Part model, mm, in its own coordinate system. A direction names the side the tool comes from. Round coordinates to 2 decimals unless told otherwise and drop trailing zeros. Loops run counter-clockwise (first coordinate to the right, second up) from the corner with the lowest first, then second, coordinate; pieces in that order, holes last. Notation, with made-up numbers: (30, 2) -> (55, 2) arc R16 cw to (55, 22) -> close; hole circle Ø3 at (3, 51.5). An arc over 180 degrees is marked (long way). Use a Markdown table: item, result. Add a question column.
Item 1: Two-plate mould, pull along Z, no slides. Class faces 3 (the face through (-16, 0, 16)), 4 (the face through (-8.94, -3.76, 20.16)), 5 (the face through (-9.996, -3.757, 2.274)): pulls with the +Z half, pulls with the -Z half, needs draft (parallel to the pull), parting line crosses it, or undercut.
Item 2: Flat gauge pins, fed straight in: pin 1 (0.6 mm diameter, centred on y = -5, z = 21.5, fed in from -X); pin 2 (2 mm diameter, centred on x = -19, y = -3.5, fed in from -Z); pin 3 (4 mm diameter, centred on x = -13.5, y = -5.5, fed in from +Z). Where does each tip first touch, or does it go through?
Item 3: Probe line 1 (X direction, y = -6, z = 18); line 2 (Z direction, x = -17.75, y = -2); line 3 (X direction, y = -5.75, z = 8.5). List the from-to ranges inside material, lowest first. Write a range as [from, to].
Item 4: Cut at C-C, the plane z = 10. List the corners of the cut face in (x, y).
Item 5: Which spindle directions (+Z, -Z, +X, -X, +Y, -Y) get a long thin tool onto all of the face, cutting with end or side? Do faces 1 (the face through (-2.32, -3.76, 9.83)), 2 (the face through (-12.346, -4, 21)). Say none if no direction does.
Item 6: Cut at D-D, the plane z = 18.25. List the corners of the cut face in (x, y), plus the area to 3 significant figures.
Item 7: Cut at B-B, the plane x = -7. List the corners of the cut face in (y, z), plus the area to 3 significant figures.
Item 8: Cut at A-A, the plane y = -2. List the corners of the cut face in (x, z).
```python
from build123d import *

# Parameters (mm, degrees)
F1_DEPTH = 7.62
F3_DEPTH = 7.62
F5_DEPTH = 7.62


with BuildPart() as f1:
    # F0 (on Front) → F1 (new body)
    with BuildSketch(Plane.XZ):
        Polygon((-0.68674681, 15.9189414907), (-9.4810585093, 24.71325319), (-21.4943116993, 21.4943116993), (-24.71325319, 9.4810585093), (-15.9189414907, 0.68674681), (-3.9056883007, 3.9056883007), align=None)
    extrude(amount=F1_DEPTH)

    # F2 (on face) → F3 (cut)
    with BuildSketch(Plane(origin=(0, 0, 0), x_dir=(-1, 0, 0), z_dir=(0, 1, 0))):
        with BuildLine():
            Line((13.7354055899, 8.8358137319), (11.6645944101, 16.5641862681))
            ThreePointArc((11.6645944101, 16.5641862681), (8.8358137319, 11.6645944101), (13.7354055899, 8.8358137319))
        make_face()
        with BuildLine():
            ThreePointArc((16.7005, 12.7), (15.1353500967, 15.8738100378), (11.6645944101, 16.5641862681))
            Line((11.6645944101, 16.5641862681), (13.7354055899, 8.8358137319))
            ThreePointArc((13.7354055899, 8.8358137319), (15.8738100378, 10.2646499033), (16.7005, 12.7))
        make_face()
    extrude(amount=-F3_DEPTH, mode=Mode.SUBTRACT)

    # F4 (on face) → F5 (cut)
    with BuildSketch(Plane(origin=(0, 0, 0), x_dir=(-1, 0, 0), z_dir=(0, 1, 0))):
        with BuildLine():
            Line((9.4810585093, 19.3075097995), (8.38471647, 21.0305488332))
            ThreePointArc((8.38471647, 21.0305488332), (3.6253777463, 10.3186250274), (13.0313017042, 3.323969124))
            Line((13.0313017042, 3.323969124), (13.1753263628, 5.3655037719))
            ThreePointArc((13.1753263628, 5.3655037719), (5.5953016242, 10.8174402904), (9.4810585093, 19.3075097995))
        make_face()
        with BuildLine():
            ThreePointArc((17.3331181487, 4.5419406703), (20.808239175, 7.9802358864), (22.0818823168, 12.7))
            ThreePointArc((22.0818823168, 12.7), (19.2078073532, 19.4578220797), (12.3464885615, 22.0752197558))
            Line((12.3464885615, 22.0752197558), (12.3464885615, 20.0413758747))
            ThreePointArc((12.3464885615, 20.0413758747), (17.7706263223, 18.0206690154), (20.0498823168, 12.7))
            ThreePointArc((20.0498823168, 12.7), (18.9642836617, 8.8555858343), (16.0281797534, 6.1468336203))
            Line((16.0281797534, 6.1468336203), (17.3331181487, 4.5419406703))
        make_face()
    extrude(amount=-F5_DEPTH, mode=Mode.SUBTRACT)


solid = f1.part
```
A:
| question | item | result |
|---|---|---|
| 1 | face 3 | needs draft |
| 1 | face 4 | undercut |
| 1 | face 5 | pulls with the -Z half |
| 2 | pin 1 | stops at x = -21.57 |
| 2 | pin 2 | stops at z = 2.77 |
| 2 | pin 3 | stops at z = 24.17 |
| 3 | line 1 | x = [-22.43, -20.44], [-17.79, -7.61], [-4.96, -2.77] |
| 3 | line 2 | z = [2.52, 4.79], [7.36, 18.04], [20.61, 22.5] |
| 3 | line 3 | x = [-23.73, -21.09], [-18.73, -6.67], [-4.31, -2.67] |
| 4 | outline | (-24.57, -7.62) -> (-21.68, -7.62) -> (-21.68, 0) -> (-24.57, 0) -> close; (-19.54, -7.62) -> (-15.65, -7.62) -> (-15.65, 0) -> (-19.54, 0) -> close; (-9.75, -7.62) -> (-5.86, -7.62) -> (-5.86, 0) -> (-9.75, 0) -> close; (-3.72, -7.62) -> (-2.27, -7.62) -> (-2.27, 0) -> (-3.72, 0) -> close |
| 5 | face 1 | -Z, +X, +Y, -Y |
| 5 | face 2 | +Y, -Y |
| 6 | outline | (-22.36, -7.62) -> (-20.26, -7.62) -> (-20.26, 0) -> (-22.36, 0) -> close; (-17.52, -7.62) -> (-7.88, -7.62) -> (-7.88, 0) -> (-17.52, 0) -> close; (-5.14, -7.62) -> (-3.02, -7.62) -> (-3.02, 0) -> (-5.14, 0) -> close |
| 6 | area | 106 mm^2 |
| 7 | outline | (-7.62, 3.08) -> (0, 3.08) -> (0, 5.25) -> (-7.62, 5.25) -> close; (-7.62, 8.06) -> (0, 8.06) -> (0, 17.34) -> (-7.62, 17.34) -> close; (-7.62, 20.15) -> (0, 20.15) -> (0, 22.23) -> (-7.62, 22.23) -> close |
| 7 | area | 103 mm^2 |
| 8 | outline | (-24.71, 9.48) -> (-15.92, 0.69) -> (-3.91, 3.91) -> (-0.69, 15.92) -> (-9.48, 24.71) -> (-21.49, 21.49) -> close; hole (-17.33, 4.54) -> (-16.03, 6.15) arc R7.35 cw to (-12.35, 20.04) -> (-12.35, 22.08) arc R9.38 ccw to start; hole circle Ø8 at (-12.7, 12.7); hole (-13.18, 5.37) -> (-13.03, 3.32) arc R9.38 ccw to (-8.38, 21.03) -> (-9.48, 19.31) arc R7.35 cw to start |
